Build history of the part. All positions in model axes, mm. Face numbers are marked on the shaded views. A direction names the side the tool comes from. Round coordinates to 2 decimals unless told otherwise and drop trailing zeros. Order: outer loops, then holes, each group sorted by start corner. A loop starts at its lowest first (then second) coordinate and runs counter-clockwise, first axis right, second up. Notation, with made-up numbers: (0.25, 60) -> (43.25, 60) arc R34 ccw to (43.25, 90) -> close; hole circle Ø5 at (12, 52). An arc over 180 degrees is marked (long way). Write item = value, one per line.
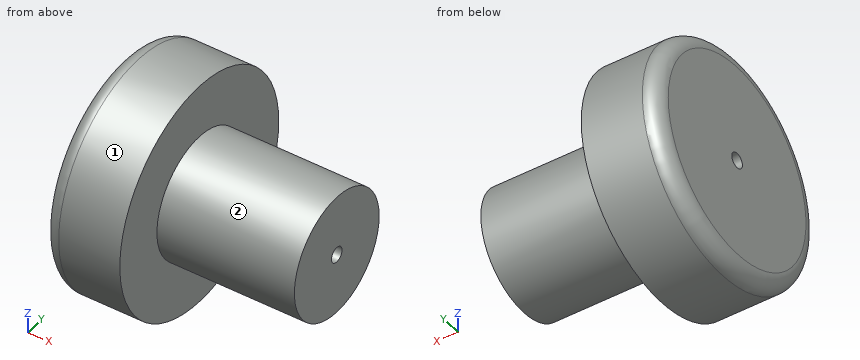
Autodesk Inventor part; units mm, degrees
ref_plane "YZ Plane" through (0, 0, 0) normal (1, 0, 0) x (0, 1, 0)
ref_plane "XZ Plane" through (0, 0, 0) normal (0, 1, 0) x (-1, 0, 0)
ref_plane "XY Plane" through (0, 0, 0) normal (0, 0, 1) x (1, 0, 0)
sketch "Skizze1" plane through (0, 0, 0) normal (0, 0, 1) x (1, 0, 0)
  line L0 (0, 0) -> (0, 7.5)
  line L1 (0, 7.5) -> (5, 7.5)
  line L2 (5, 7.5) -> (5, 4)
  line L3 (5, 4) -> (14, 4)
  line L4 (14, 4) -> (14, 0)
  line L5 (14, 0) -> (0, 0)
  dimension "d0" = 15
  dimension "d1" = 9
  dimension "d2" = 5
  dimension "d3" = 8
revolve "Umdrehung1" add sketch "Skizze1" angle 360 about axis through (14, 0, 0) along (-1, 0, 0)
thread "Gewinde1"
sketch "Skizze2" plane through (0, 0, 0) normal (-1, 0, 0) x (0, 0, 1)
  circle A0 centre (0, 0) radius 7.5
  point P0 (0, 0)
hole "Bohrung1" at (0, 0, 0) direction (1, 0, 0) diameter 1 depth 14
fillet "Rundung1" radius 1 1 edges at (0, -7.5, 0)
properties part number "1 part 4" material "Stahl, galvanisiert"
Q1. Cut at D-D, the plane x = 2.25. List the corners of the cut face in (y, z).
Check values:
outline = circle Ø15 at (0, 0); hole circle Ø1 at (0, 0)
Q2. Cut at A-A, the plane y = 0. List the corners of the cut face in (x, z).
Check values:
outline = (0, -6.5) arc R1 ccw to (1, -7.5) -> (5, -7.5) -> (5, -4) -> (14, -4) -> (14, -0.5) -> (0, -0.5) -> close; (0, 0.5) -> (14, 0.5) -> (14, 4) -> (5, 4) -> (5, 7.5) -> (1, 7.5) arc R1 ccw to (0, 6.5) -> close
Q3. Flat gauge pin, fed straight in: pin 1 (2 mm diameter, centred on x = 11, y = -3.5, fed in from +Z). Where does the tip first touch, or does it go through?
Check values:
pin_1 = 3.12
Q4. Cut at C-C, the plane x = 6.75. List the corners of the cut face in (y, z).
Check values:
outline = circle Ø8 at (0, 0); hole circle Ø1 at (0, 0)
Q5. Which spindle directions (+Z, -Z, +X, -X, +Y, -Y) get a long thin tool onto all of the face, cutting with end or side? Do the marked faces 1 and 2. Say none if no direction does.
Check values:
face_1 = +X, -X
face_2 = +X
Q6. Probe probe 1 along Z at (x, y) = (3, 0); probe 2 along Z at (x, y) = (5.25, 0); probe 3 along X at (y, z) = (-5.5, -0.25). List the from-to ranges inside material, lowest first.
Check values:
probe_1 = -7.5 to -0.5, 0.5 to 7.5
probe_2 = -4 to -0.5, 0.5 to 4
probe_3 = 0 to 5
